Verification items for the finished model (mm, model axes). A direction names the side the tool comes from. Coordinates: 2 decimals unless noted, no trailing zeros. Answer in a Markdown table with one row per item.
```python
from build123d import *

# Parameters (mm, degrees)
F0_W           = 107.95
F0_H           = 181.61
F1_DEPTH       = 3.175
F3_D           = 3.7973
F3_CSINK_D     = 7.7978
F3_CSINK_ANGLE = 82
F4_R           = 5.08
F5_W           = 12.7
F5_H           = 12.7
F6_DEPTH       = 0.127


with BuildPart() as f1:
    # F0 (on Top) → F1 (new body)
    with BuildSketch(Plane.XY):
        with Locations((53.975, 90.805)):
            Rectangle(F0_W, F0_H)
    extrude(amount=F1_DEPTH)

    # F3 (through all)
    with Locations(Plane(origin=(0, 0, 0), x_dir=(1, 0, 0), z_dir=(0, 0, -1))):
        with Locations((8.255, -8.255), (99.695, -8.255), (99.695, -80.645), (8.255, -80.645), (8.255, -100.965), (8.255, -173.355), (99.695, -173.355), (99.695, -100.965)):
            CounterSinkHole(F3_D / 2, F3_CSINK_D / 2, counter_sink_angle=F3_CSINK_ANGLE)

    # F4
    f4_edges = [f1.edges().sort_by_distance(p)[0] for p in [
        (0, 0, 1.5875),
        (107.95, 0, 1.5875),
        (107.95, 181.61, 1.5875),
        (0, 181.61, 1.5875),
    ]]
    fillet(f4_edges, radius=F4_R)

    # F5 (on face) → F6 (cut)
    with BuildSketch(Plane(origin=(0, 0, 0), x_dir=(1, 0, 0), z_dir=(0, 0, -1))):
        with Locations((19.05, -19.05)):
            Rectangle(F5_W, F5_H)
        with Locations((88.9, -19.05)):
            Rectangle(F5_W, F5_H)
        with Locations((19.05, -162.56)):
            Rectangle(F5_W, F5_H)
        with Locations((88.9, -162.56)):
            Rectangle(F5_W, F5_H)
    extrude(amount=-F6_DEPTH, mode=Mode.SUBTRACT)


solid = f1.part
```
1. Release check for a two-part mould opening along X. For faces 1 (the face through (106.501, 1.528, 1.61)), 2 (the face through (1.449, 1.528, 1.61)), 3 (the face through (101.094, 6.972, 2.744)) record: released by +X, released by -X, zero draft, split by the parting line, or undercut.
Findings below:
| item | result |
|---|---|
| face 1 | released by +X |
| face 2 | released by -X |
| face 3 | undercut |
2. Access from +Z, -Z, +X, -X, +Y, -Y to the whole of each face (thin tool, end or side, straight path). Record for faces 4 (the face through (107.95, 90, 2)), 5 (the face through (19, 19, 0.127)).
Findings below:
| item | result |
|---|---|
| face 4 | +Z, -Z, +X, +Y, -Y |
| face 5 | -Z |
3. Sectioned sample at A-A, the plane z = 0.65. Count the separate pieces of the cut face and the enclosed holes in it, and give its area (3 significant figures).
Findings below:
| item | result |
|---|---|
| separate pieces | 1 |
| enclosed holes | 8 |
| area | 19,300 mm² |
4. Go/stop test with flat-tipped pins: pin 1 (10 mm diameter, centred on x = 19.5, y = 19, fed in from -Z); pin 2 (5 mm diameter, centred on x = 99.695, y = 100.965, fed in from -Z). Record where each tip stops, or that it passes through.
Findings below:
| item | result |
|---|---|
| pin 1 | stops at z = 0.13 |
| pin 2 | stops at z = 1.61 |
